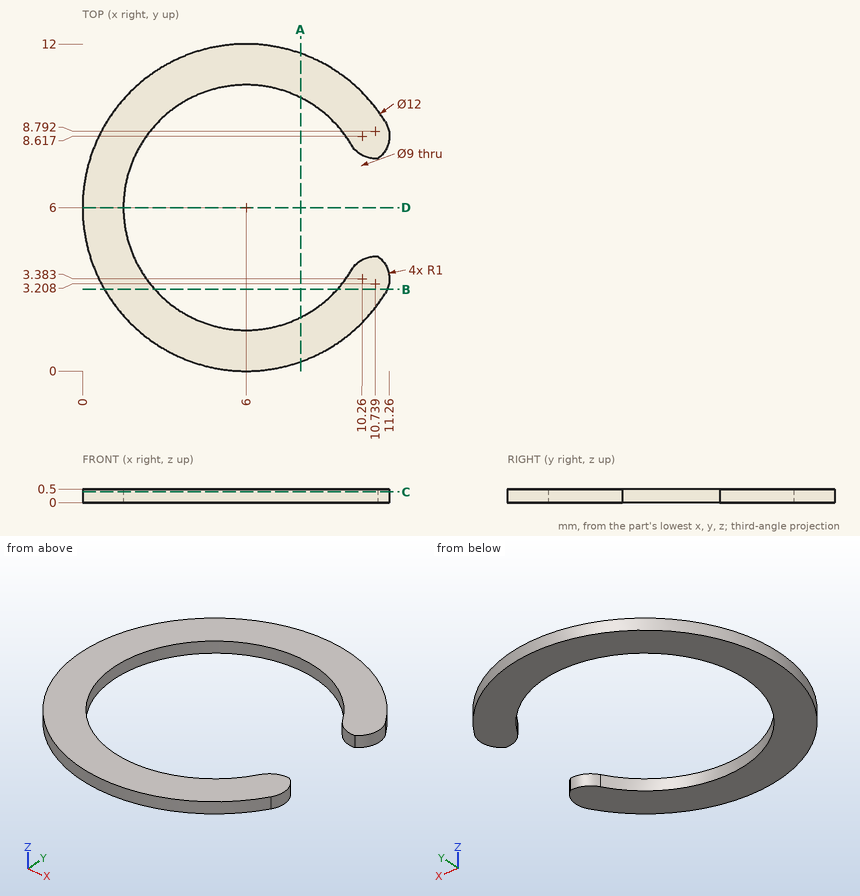
Geometry: see drawing. Coordinates: mm, zero at the bounding-box minimum. Coordinates: 2 decimals unless noted, no trailing zeros. Order: outer loops, then holes, each group sorted by start corner. A loop starts at its lowest first (then second) coordinate and runs counter-clockwise, first axis right, second up. Notation, with made-up numbers: M 40.25,-33.5 L 63.25,-33.5 A14 ccw 63.25,-27.5 Z; hole C 44,-14.5 d8. An arc over 180 degrees is marked long. Write item = value, one per line. Start each with the question number.
(1) Section A-A on x = 8. Output: boundary loops of the cut face in (y, z).
(2) First-contact query: P1, Ø2, axis at x = 7, y = 1.5, coming from the -Z side; P2, Ø3, axis at x = 7, y = 3.5, coming from the +Z side. Flat tips, straight axial feed; report the tip coordinate or a pass-through.
(3) Section C-C on z = 0.4. Output: boundary loops of the cut face in (x, y).
(4) Line query: line 1 along Y through (x, z) = (6, 0.35); line 2 along X through (y, z) = (6, 0.4); line 3 along X through (y, z) = (3, 0.15) (1 decimal). Output: solid intervals per line, ascending. Write a range as [from, to].
(5) Section D-D on y = 6. Output: boundary loops of the cut face in (x, z).
(6) Section B-B on y = 3. Output: boundary loops of the cut face in (x, z).
Result set:
q1.outline = M 0.34,0 L 1.97,0 L 1.97,0.5 L 0.34,0.5 Z; M 10.03,0 L 11.66,0 L 11.66,0.5 L 10.03,0.5 Z
q2.P1 = 0
q2.P2 = through
q3.outline = M 9.88,3.72 A4.5 cw long 9.88,8.28 A1 ccw 10.83,7.8 A1 ccw 11.11,9.14 A6 ccw long 11.11,2.86 A1 ccw 10.83,4.2 A1 ccw Z
q4.line_1 = [0, 1.5], [10.5, 12]
q4.line_2 = [0, 1.5]
q4.line_3 = [0.8, 2.6], [9.4, 11.2]
q5.outline = M 0,0 L 1.5,0 L 1.5,0.5 L 0,0.5 Z
q6.outline = M 0.8,0 L 2.65,0 L 2.65,0.5 L 0.8,0.5 Z; M 9.35,0 L 11.18,0 L 11.18,0.5 L 9.35,0.5 Z
